Check sheet for the modelled part. Datum: model origin and axes. Units: mm. A direction names the side the tool comes from. Round coordinates to 2 decimals unless told otherwise and drop trailing zeros. Write each loop counter-clockwise with the first axis right and the second up, starting at its lowest first coordinate (ties: lowest second). Pieces come first, ordered by that corner, then holes. Notation, with made-up numbers: (-36, 46) - (21, 46) arc R21 cw to (21, 66) - close; hole circle Ø1 at (20, 56). An arc over 180 degrees is marked (long way). Use one line per item in the form item = value. Start each with the question number.
1) Section check A-A (z = 0.8). Record the boundary of the cut face in (x, y), then the cut area to 3 significant figures.
2) Gauge pin test, flat ends, axial feed: P1, Ø1, axis at x = -72, z = 1.5, coming from the -Y side; P2, Ø1, axis at x = -71.5, z = 1, coming from the +Y side; P3, Ø1.6, axis at y = -0.5, z = 1, coming from the -X side. Record the tip position at first contact, or that the pin passes through.
3) Scan lines: probe 1 along Z at (x, y) = (14, -56); probe 2 along X at (y, z) = (-2, 1.9); probe 3 along Y at (x, z) = (-66, 1.4). Record each from-to range of solid material in increasing order.
4) Draft check along Y on faces 1 (the face through (-60.6, -55.9, 1)), 2 (the face through (-60.9, 55.6, 1)), 3 (the face through (49, 1, 2)). Enter one of: +Y half, -Y half, draft (parallel to the pull), parting line (faces both ways), or undercut.
5) Section check C-C (x = -3.16). Record the boundary of the cut face in (y, z).
6) Set-up check for faces 4 (the face through (44.53, 15.02, 2.49)), 5 (the face through (-21.533, 62.743, 1.014)): record each of +Z, -Z, +X, -X, +Y, -Y from which the full face is reachable in a straight line by a thin tool's end or side.
7) Section check D-D (y = 54). Record the boundary of the cut face in (x, z).
8) Section check B-B (y = 0). Record the boundary of the cut face in (x, z), then the cut area to 3 significant figures.
from build123d import *

# Parameters (mm, degrees)
F0_W     = 150
F0_H     = 140
F1_DEPTH = 2
F3_DEPTH = 2.001
F5_DEPTH = 2.001
F7_DEPTH = 2.001
F8_R     = 50
F9_DEPTH = 1


with BuildPart() as f1:
    # F0 (on Top) → F1 (new body)
    with BuildSketch(Plane.XY):
        Rectangle(F0_W, F0_H)
    extrude(amount=F1_DEPTH)

    # F2 (on face) → F3 (cut, through all)
    with BuildSketch(Plane.XY.offset(2)):
        Polygon((-75, 70), (-75, 41.5), (-46.5, 70), align=None)
        Polygon((-46.5, -70), (-75, -41.5), (-75, -70), align=None)
    extrude(amount=-F3_DEPTH, mode=Mode.SUBTRACT)

    # F4 (on face) → F5 (cut, through all)
    with BuildSketch(Plane.XY.offset(2)):
        with BuildLine():
            Line((-69.68, 9.5), (-75, 9.5))
            Line((-75, 9.5), (-75, -9.5))
            Line((-75, -9.5), (-69.68, -9.5))
            ThreePointArc((-69.68, -9.5), (-67.912233, -8.767767), (-67.18, -7))
            Line((-67.18, -7), (-67.18, 7))
            ThreePointArc((-67.18, 7), (-67.912233, 8.767767), (-69.68, 9.5))
        make_face()
    extrude(amount=-F5_DEPTH, mode=Mode.SUBTRACT)

    # F6 (on face) → F7 (cut, through all)
    with BuildSketch(Plane.XY.offset(2)):
        with BuildLine():
            Line((-28.031671, -70), (-15, -70))
            Line((-15, -70), (-16.416769, -66.495551))
            ThreePointArc((-16.416769, -66.495551), (-21.515836, -63.056988), (-26.614902, -66.495551))
            Line((-26.614902, -66.495551), (-28.031671, -70))
        make_face()
        with BuildLine():
            Line((-27.876137, 70), (-26.631231, 66.430881))
            ThreePointArc((-26.631231, 66.430881), (-21.438069, 62.742254), (-16.244907, 66.430881))
            Line((-16.244907, 66.430881), (-15, 70))
            Line((-15, 70), (-27.876137, 70))
        make_face()
    extrude(amount=-F7_DEPTH, mode=Mode.SUBTRACT)

    # F8 (on face) → F9 (join)
    with BuildSketch(Plane.XY.offset(2)):
        with Locations((-3.16, 0)):
            Circle(F8_R)
    extrude(amount=F9_DEPTH)


solid = f1.part
Results are:
q1.outline = (-75, -41.5) - (-46.5, -70) - (-28.03, -70) - (-26.61, -66.5) arc R5.5 cw to (-16.42, -66.5) - (-15, -70) - (75, -70) - (75, 70) - (-15, 70) - (-16.24, 66.43) arc R5.5 cw to (-26.63, 66.43) - (-27.88, 70) - (-46.5, 70) - (-75, 41.5) - (-75, 9.5) - (-69.68, 9.5) arc R2.5 cw to (-67.18, 7) - (-67.18, -7) arc R2.5 cw to (-69.68, -9.5) - (-75, -9.5) - close
q1.area = 19,900 mm²
q2.P1 = -45
q2.P2 = 45.5
q2.P3 = -67.18
q3.probe_1 = 0 to 2
q3.probe_2 = -67.18 to 75
q3.probe_3 = -50.5 to 50.5
q4.face_1 = -Y half
q4.face_2 = +Y half
q4.face_3 = draft
q5.outline = (-70, 0) - (70, 0) - (70, 2) - (50, 2) - (50, 3) - (-50, 3) - (-50, 2) - (-70, 2) - close
q6.face_4 = +Z
q6.face_5 = +Z, -Z, +Y
q7.outline = (-62.5, 0) - (75, 0) - (75, 2) - (-62.5, 2) - close
q8.outline = (-67.18, 0) - (75, 0) - (75, 2) - (46.84, 2) - (46.84, 3) - (-53.16, 3) - (-53.16, 2) - (-67.18, 2) - close
q8.area = 384 mm²
